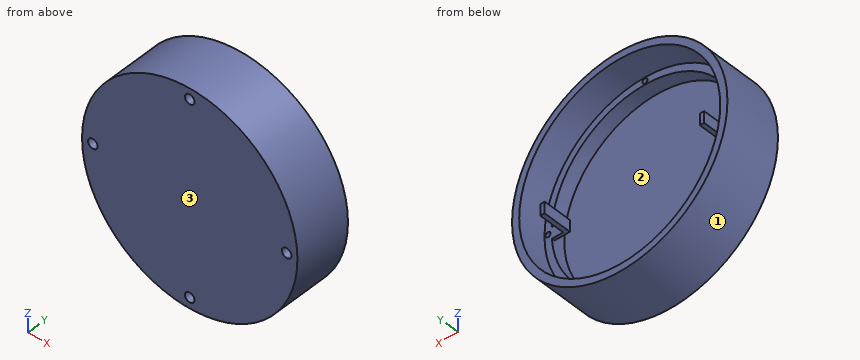
Autodesk Inventor part; units mm, degrees
ref_plane "작업 평면1" through (57, 0, 0) normal (1, 0, 0) x (0, 1, 0)
ref_plane "XZ Plane" through (0, 0, 0) normal (0, 1, 0) x (-1, 0, 0)
ref_plane "XY Plane" through (0, 0, 0) normal (0, 0, 1) x (1, 0, 0)
sketch "스케치1" plane through (0, 0, 0) normal (0, 1, 0) x (-1, 0, 0)
  circle A0 centre (0, 0) radius 75
  dimension "d0" = 150
extrude "돌출1" add sketch "스케치1" along normal blind 40
shell "쉘1" thickness 10 removed faces 1 at (17.2828, 40, 11.7077)
sketch "스케치6" plane through (0, 40, 0) normal (0, 1, 0) x (1, 0, 0)
  circle A0 centre (0, 0) radius 65
  circle A1 centre (0, 0) radius 70
  dimension "d22" = 130
  dimension "d23" = 140
extrude "돌출5" cut sketch "스케치6" against normal blind 20
sketch "스케치8" plane through (0, 0, 0) normal (0, -1, 0) x (1, 0, 0)
  circle A0 centre (0, 0) radius 67.5
  point P0 (0, -67.5)
  point P1 (67.5, 0)
  point P2 (0, 67.5)
  point P3 (-67.5, 0)
  dimension "d31" = 135
hole "구멍2" at (0, 0, -67.5) at (67.5, 0, 0) at (0, 0, 67.5) at (-67.5, 0, 0) direction (0, 1, 0) diameter 3.5 depth 25 counterbore diameter 6.7 counterbore depth 9
ref_plane "작업 평면1" through (57, 0, 0) normal (1, 0, 0) x (0, 1, 0)
sketch "스케치10" plane through (57, 0, 0) normal (1, 0, 0) x (0, 1, 0)
  line L0 (38, -4.2173) -> (18, -4.2173)
  line L1 (18, -4.2173) -> (18, 3.7827)
  line L2 (18, 3.7827) -> (38, 3.7827)
  line L3 (38, 3.7827) -> (38, -4.2173)
  line L4 (38, -4.2173) -> (18, 3.7827) construction
  line L5 (18, -4.2173) -> (38, 3.7827) construction
  line L6 (10, 65) -> (10, -65)
  point P0 (0, 0)
  point P1 (28, -0.2173)
  dimension "d40" = 20
  dimension "d41" = 8
  dimension "d42" = 18
extrude "돌출6" add sketch "스케치10" against normal blind 3
sketch "스케치11" plane through (57, 0, 0) normal (1, 0, 0) x (0, 0, -1)
  line L0 (4.2173, 38) -> (4.2173, 18)
  line L1 (4.2173, 18) -> (-3.7827, 18)
  line L2 (-3.7827, 18) -> (-3.7827, 20)
  line L3 (-3.7827, 20) -> (4.2173, 20)
  line L4 (4.2173, 20) -> (4.2173, 18)
  point P0 (0, 0)
  dimension "d45" = 8
  dimension "d46" = 2
extrude "돌출7" add sketch "스케치11" along normal up to next
pattern_circular "원형 패턴1" count 2 over 360 about axis through (0, 0, 0) along (0, 1, 0) of "돌출6", "돌출7"
properties part number "바텀(하)"
Here's how the part is built. I have some questions about the finished solid (model axes, mm). Face numbers are marked on the shaded views. Coordinates: 2 decimals unless noted, no trailing zeros. Write each loop counter-clockwise with the first axis right and the second up, starting at its lowest first coordinate (ties: lowest second). Pieces come first, ordered by that corner, then holes. Notation, with made-up numbers: (-25.75, 87) - (25.25, 87) arc R12 ccw to (25.25, 106) - close; hole circle Ø3 at (55, 58). An arc over 180 degrees is marked (long way). Use one line per item in the form item = value.
1) Thinking about a two-plate mould opening in X: for the marked faces 1, 2 and 3, which applies, released by +X, released by -X, zero draft, split by the parting line, or undercut?
Solved:
face_1 = split by the parting line
face_2 = undercut
face_3 = zero draft
2) Suppose I cut it at A-A, the plane y = 31. Write out the boundary of the cut face in (x, z), plus the area to 3 significant figures.
Solved:
outline = circle Ø150 at (0, 0); (-57, -3.78) - (-54, -3.78) - (-54, 4.22) - (-57, 4.22) - close; (54, -4.22) - (57, -4.22) - (57, 3.78) - (54, 3.78) - close; hole circle Ø140 at (0, 0)
area = 2,330 mm2
3) I'm going to push flat-ended pins straight in: P1, Ø5, axis at y = 36, z = -36, coming from the +X side; P2, Ø2, axis at x = -68.5, z = 0, coming from the -Y side; P3, Ø6, axis at x = 14, y = 9.5, coming from the +Z side; P4, Ø4, axis at x = 59.5, z = 1, coming from the -Y side. Where does each tip first touch, or does it pass through?
Solved:
P1 = 67.1
P2 = 9
P3 = 74.19
P4 = 0
4) Suppose I cut it at C-C, the plane z = 67.5. Write out the boundary of the cut face in (x, y), plus the area to 3 significant figures.
Solved:
outline = (-32.69, 0) - (-3.35, 0) - (-3.35, 9) - (-1.75, 9) - (-1.75, 20) - (-18.54, 20) - (-18.54, 40) - (-32.69, 40) - close; (1.75, 9) - (3.35, 9) - (3.35, 0) - (32.69, 0) - (32.69, 40) - (18.54, 40) - (18.54, 20) - (1.75, 20) - close
area = 1,770 mm2
5) Suppose I cut it at B-B, the plane x = -67.5. Write out the boundary of the cut face in (y, z).
Solved:
outline = (0, -32.69) - (40, -32.69) - (40, -18.54) - (20, -18.54) - (20, -1.75) - (9, -1.75) - (9, -3.35) - (0, -3.35) - close; (0, 3.35) - (9, 3.35) - (9, 1.75) - (20, 1.75) - (20, 18.54) - (40, 18.54) - (40, 32.69) - (0, 32.69) - close
6) Suppose I cut it at D-D, the plane y = 15.5. Write out the boundary of the cut face in (x, z).
Solved:
outline = circle Ø150 at (0, 0); hole circle Ø3.5 at (-67.5, 0); hole circle Ø130 at (0, 0); hole circle Ø3.5 at (0, -67.5); hole circle Ø3.5 at (0, 67.5); hole circle Ø3.5 at (67.5, 0)
7) I need wall thicknesses on line 1 (Z direction, x = 0, y = 14.25); line 2 (Z direction, x = 1.5, y = 7.5) (3 decimals); line 3 (Y direction, x = 7, z = -19). Which ranges of each line are inside material? Lowest first, please.
Solved:
line_1 = -75 to -69.25, -65.75 to -65, 65 to 65.75, 69.25 to 75
line_2 = -74.985 to -70.495, -64.505 to 64.505, 70.495 to 74.985
line_3 = 0 to 10
